The listing builds one solid part. Answer for the finished solid, in the listing's coordinates (mm). A direction names the side the tool comes from. Round coordinates to 2 decimals unless told otherwise and drop trailing zeros. Order: outer loops, then holes, each group sorted by start corner. A loop starts at its lowest first (then second) coordinate and runs counter-clockwise, first axis right, second up. Notation, with made-up numbers: (47.25, -30.75) -> (103.25, -30.75) arc R19 ccw to (103.25, -14.75) -> close; hole circle Ø10 at (27.25, -19.75). An arc over 180 degrees is marked (long way). Answer in a Markdown table with one row per item. Add a question column.
```python
from build123d import *

# Parameters (mm, degrees)
SKETCH_1_R          = 7.5
EXTRUDE_1_DEPTH     = 9.5
SKETCH_2_R          = 10
CUT_EXTRUDE_1_DEPTH = 6


with BuildPart() as part:
    # 草图1 → 凸台-拉伸1 (new body)
    with BuildSketch(Plane(origin=(0, 0, 0), x_dir=(1, 0, 0), z_dir=(0, 1, 0))):
        Polygon((-8, 14), (8, 14), (8, 8), (14, 8), (14, -8), (8, -8), (8, -14), (-8, -14), (-8, -8), (-14, -8), (-14, 8), (-8, 8), align=None)
        Circle(SKETCH_1_R, mode=Mode.SUBTRACT)
    extrude(amount=EXTRUDE_1_DEPTH)

    # 草图2 → 切除-拉伸1 (cut)
    with BuildSketch(Plane.XZ):
        Circle(SKETCH_2_R)
    extrude(amount=-CUT_EXTRUDE_1_DEPTH, mode=Mode.SUBTRACT)


solid = part.part
```
Item 1: Find the intervals of material crossed by probe 1 along X at (y, z) = (7.3, 0); probe 2 along Z at (x, y) = (6, 1); probe 3 along X at (y, z) = (9.25, -9.5), in increasing order. Write a range as [from, to].
Item 2: The part is cut by section C-C, the plane x = 10.75. Give the vertices of the cut face in (y, z).
Item 3: The part is cut by section B-B, the plane z = 0. Give the vertices of the cut face in (x, y), and give its area (3 significant figures).
Item 4: Flat-ended cylindrical pins translate along their axes: P1, Ø3, axis at x = 11.5, y = 5.5, coming from the +Z side; P2, Ø5, axis at y = 3, z = 11, coming from the -X side. Find the tip coordinate at first contact, or state that the pin passes through.
Item 5: A tool of negligible diameter and unlimited length cuts with its end or side. For faces 5 (the face through (-8, 5, 11)), 6 (the face through (11, 5, -8)), 7 (the face through (-8, 5, -11)), from which of +Z, -Z, +X, -X, +Y, -Y can it reach the whole face along a straight path? Write none if from no direction.
Item 6: For a pull along X with two mould halves and no side action, classify faces 1 (the face through (-2.17, 2.96, -9.76)), 2 (the face through (14, 5, 0)), 3 (the face through (-7.493, 7.726, -0.33)), 4 (the face through (-11, 5, -8)) as released by +X, released by -X, zero draft, split by the parting line, or undercut.
Item 7: The part is cut by section A-A, the plane x = 0. Give the vertices of the cut face in (y, z), and give its area (3 significant figures).
Resolved:
| question | item | result |
|---|---|---|
| 1 | probe 1 | [-14, -7.5], [7.5, 14] |
| 1 | probe 2 | [-14, -8], [8, 14] |
| 1 | probe 3 | [-8, 8] |
| 2 | outline | (0, -8) -> (9.5, -8) -> (9.5, 8) -> (0, 8) -> close |
| 3 | outline | (-14, 0) -> (-10, 0) -> (-10, 6) -> (-7.5, 6) -> (-7.5, 9.5) -> (-14, 9.5) -> close; (7.5, 6) -> (10, 6) -> (10, 0) -> (14, 0) -> (14, 9.5) -> (7.5, 9.5) -> close |
| 3 | area | 93.5 mm2 |
| 4 | P1 | z = 8 |
| 4 | P2 | x = -8 |
| 5 | face 5 | +Z, -X, +Y, -Y |
| 5 | face 6 | -Z, +X, +Y, -Y |
| 5 | face 7 | -Z, -X, +Y, -Y |
| 6 | face 1 | undercut |
| 6 | face 2 | released by +X |
| 6 | face 3 | undercut |
| 6 | face 4 | zero draft |
| 7 | outline | (0, -14) -> (9.5, -14) -> (9.5, -7.5) -> (6, -7.5) -> (6, -10) -> (0, -10) -> close; (0, 10) -> (6, 10) -> (6, 7.5) -> (9.5, 7.5) -> (9.5, 14) -> (0, 14) -> close |
| 7 | area | 93.5 mm2 |
